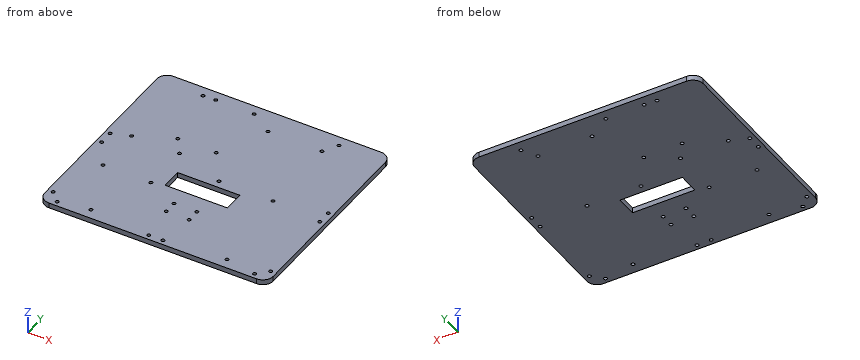
```python
from build123d import *

# Parameters (mm, degrees)
MODEL_R         = 1.65
MODEL_W         = 60
MODEL_H         = 20
EXTRUDE_1_DEPTH = 5


with BuildPart() as part:
    # Model → 凸台-拉伸1 (new body)
    with BuildSketch(Plane.XY):
        with BuildLine():
            Line((196.361294225, 321.408553495), (396.361294225, 321.408553495))
            ThreePointArc((396.361294225, 321.408553495), (403.432362037, 318.479621307), (406.361294225, 311.408553495))
            Line((406.361294225, 311.408553495), (406.361294225, 131.408553495))
            ThreePointArc((406.361294225, 131.408553495), (403.432362037, 124.337485683), (396.361294225, 121.408553495))
            Line((396.361294225, 121.408553495), (196.361294225, 121.408553495))
            ThreePointArc((196.361294225, 121.408553495), (189.290226413, 124.337485683), (186.361294225, 131.408553495))
            Line((186.361294225, 131.408553495), (186.361294225, 311.408553495))
            ThreePointArc((186.361294225, 311.408553495), (189.290226413, 318.479621307), (196.361294225, 321.408553495))
        make_face()
        with Locations((230.861294225, 311.408553495)):
            Circle(MODEL_R, mode=Mode.SUBTRACT)
        with Locations((361.861294225, 311.408553495)):
            Circle(MODEL_R, mode=Mode.SUBTRACT)
        with Locations((230.861294225, 131.408553495)):
            Circle(MODEL_R, mode=Mode.SUBTRACT)
        with Locations((361.861294225, 131.408553495)):
            Circle(MODEL_R, mode=Mode.SUBTRACT)
        with Locations((279.861294225, 311.908553495)):
            Circle(MODEL_R, mode=Mode.SUBTRACT)
        with Locations((279.861294225, 250.908553495)):
            Circle(MODEL_R, mode=Mode.SUBTRACT)
        with Locations((242.861294225, 311.908553495)):
            Circle(MODEL_R, mode=Mode.SUBTRACT)
        with Locations((242.861294225, 250.908553495)):
            Circle(MODEL_R, mode=Mode.SUBTRACT)
        with Locations((208.361294225, 234.408553495)):
            Circle(MODEL_R, mode=Mode.SUBTRACT)
        with Locations((254.361294225, 234.408553495)):
            Circle(MODEL_R, mode=Mode.SUBTRACT)
        with Locations((208.361294225, 188.408553495)):
            Circle(MODEL_R, mode=Mode.SUBTRACT)
        with Locations((254.361294225, 188.408553495)):
            Circle(MODEL_R, mode=Mode.SUBTRACT)
        with Locations((301.761294225, 297.408553495)):
            Circle(MODEL_R, mode=Mode.SUBTRACT)
        with Locations((301.761294225, 218.808553495)):
            Circle(MODEL_R, mode=Mode.SUBTRACT)
        with Locations((353.761294225, 297.408553495)):
            Circle(MODEL_R, mode=Mode.SUBTRACT)
        with Locations((353.761294225, 218.808553495)):
            Circle(MODEL_R, mode=Mode.SUBTRACT)
        with Locations((201.361294225, 126.408553495)):
            Circle(MODEL_R, mode=Mode.SUBTRACT)
        with Locations((191.673931322, 136.095916397)):
            Circle(MODEL_R, mode=Mode.SUBTRACT)
        with Locations((391.361294225, 126.408553495)):
            Circle(MODEL_R, mode=Mode.SUBTRACT)
        with Locations((401.048657127, 136.095916397)):
            Circle(MODEL_R, mode=Mode.SUBTRACT)
        with Locations((289.511294225, 126.408553495)):
            Circle(MODEL_R, mode=Mode.SUBTRACT)
        with Locations((303.211294225, 126.408553495)):
            Circle(MODEL_R, mode=Mode.SUBTRACT)
        with Locations((401.361294225, 228.258553495)):
            Circle(MODEL_R, mode=Mode.SUBTRACT)
        with Locations((401.361294225, 214.558553495)):
            Circle(MODEL_R, mode=Mode.SUBTRACT)
        with Locations((191.361294225, 228.258553495)):
            Circle(MODEL_R, mode=Mode.SUBTRACT)
        with Locations((191.361294225, 214.558553495)):
            Circle(MODEL_R, mode=Mode.SUBTRACT)
        with Locations((285.361294225, 173.908553495)):
            Circle(MODEL_R, mode=Mode.SUBTRACT)
        with Locations((307.361294225, 173.908553495)):
            Circle(MODEL_R, mode=Mode.SUBTRACT)
        with Locations((285.361294225, 161.408553495)):
            Circle(MODEL_R, mode=Mode.SUBTRACT)
        with Locations((307.361294225, 161.408553495)):
            Circle(MODEL_R, mode=Mode.SUBTRACT)
        with Locations((296.361294225, 201.408553495)):
            Rectangle(MODEL_W, MODEL_H, mode=Mode.SUBTRACT)
    extrude(amount=EXTRUDE_1_DEPTH)


solid = part.part
```
Build history of the part. All positions in model axes, mm. Coordinates: 2 decimals unless noted, no trailing zeros. Write each loop counter-clockwise with the first axis right and the second up, starting at its lowest first coordinate (ties: lowest second). Pieces come first, ordered by that corner, then holes.
1. Band-saw the part on A-A, the plane x = 320.5. Give the cut face in (y, z).
Answer block:
outline: (121.41, 0) - (191.41, 0) - (191.41, 5) - (121.41, 5) - close; (211.41, 0) - (321.41, 0) - (321.41, 5) - (211.41, 5) - close
2. Drill centre lines: probe 1 along X at (y, z) = (251, 4.05); probe 2 along Y at (x, z) = (293, 3.9); probe 3 along X at (y, z) = (228, 3.9). Where is each one in solid material? Low to high.
Answer block:
probe 1: x = 186.36 to 241.21, 244.51 to 278.21, 281.51 to 406.36
probe 2: y = 121.41 to 191.41, 211.41 to 321.41
probe 3: x = 186.36 to 189.73, 192.99 to 399.73, 402.99 to 406.36
3. Drop a flat-ended pin along its axis: pin 1 (3 mm diameter, centred on x = 353.76, y = 218.81, fed in from +Z). Give the stop position or say it passes through.
Answer block:
pin 1: passes through
4. Band-saw the part on C-C, the plane z = 3.6. Give the number of separate pieces and of enclosed holes in the cut face, and give its area (3 significant figures).
Answer block:
separate pieces: 1
enclosed holes: 31
area: 42,500 mm2
5. Band-saw the part on B-B, the plane y = 197.5. Give the cut face in (x, z).
Answer block:
outline: (186.36, 0) - (266.36, 0) - (266.36, 5) - (186.36, 5) - close; (326.36, 0) - (406.36, 0) - (406.36, 5) - (326.36, 5) - close
